Autodesk Fusion 360 part; units mm, degrees
sketch "Skizze1" plane through (0, 0, 0) normal (0, 1, 0) x (1, 0, 0)
  circle A0 centre (0, 0) radius 7.1
  dimension "d1" = 14.2
extrude "Extrusion1" add sketch "Skizze1" along normal blind 50.2

Autodesk Fusion 360 part; units mm, degrees
sketch "Skizze1" plane through (0, 0, 0) normal (0, 1, 0) x (1, 0, 0)
  line L0 (-14.5, 9) -> (14.5, 9)
  line L1 (14.5, 9) -> (14.5, -9)
  line L2 (14.5, -9) -> (-14.5, -9)
  line L3 (-14.5, -9) -> (-14.5, 9)
  line L4 (0, 0) -> (0, 9) construction
  line L5 (0, 0) -> (14.5, 0) construction
  dimension "d1" = 29
  dimension "d2" = 18
extrude "Extrusion1" add sketch "Skizze1" along normal blind 4

Autodesk Fusion 360 part; units mm, degrees
sketch "Skizze1" plane through (0, 0, 0) normal (0, 1, 0) x (1, 0, 0)
  line L0 (-15.015, 0) -> (31.025, 0) construction
  line L1 (-15.015, 0) -> (-15.015, -7.62)
  line L2 (-15.015, -7.62) -> (15.015, -7.62)
  line L3 (15.015, -7.62) -> (16.625, -6.01)
  line L4 (16.625, -6.01) -> (31.025, -6.01)
  line L5 (31.025, -6.01) -> (31.025, 0)
  line L6 (-15.015, 0) -> (-15.015, 7.62)
  line L7 (-15.015, 7.62) -> (15.015, 7.62)
  line L8 (15.015, 7.62) -> (16.625, 6.01)
  line L9 (16.625, 6.01) -> (31.025, 6.01)
  line L10 (31.025, 6.01) -> (31.025, 0)
  line L11 (0, 0) -> (0, 7.62) construction
  dimension "d1" = 12.02
  dimension "d2" = 15.24
  dimension "d3" = 30.03
  dimension "d4" = 14.4
  dimension "d5" = 46.04
extrude "Extrusion1" add sketch "Skizze1" along normal blind 3

Autodesk Fusion 360 part; units mm, degrees
sketch "Skizze1" plane through (0, 0, 0) normal (0, 1, 0) x (1, 0, 0)
  line L0 (-17, 17) -> (17, 17)
  line L1 (17, 17) -> (17, -17)
  line L2 (17, -17) -> (-17, -17)
  line L3 (-17, -17) -> (-17, 17)
  line L4 (0, 0) -> (0, 17) construction
  line L5 (0, 0) -> (17, 0) construction
  circle A0 centre (0, 0) radius 2
  circle A1 centre (-14, 14) radius 1.55
  circle A2 centre (14, 14) radius 1.55
  circle A3 centre (-14, -14) radius 1.55
  circle A4 centre (14, -14) radius 1.55
  circle A5 centre (0, 0) radius 5
  circle A6 centre (-13.25, -7.5) radius 1.25
  line L6 (-12, -7.5) -> (-12, 7.5)
  line L7 (-14.5, -7.5) -> (-14.5, 7.5)
  circle A7 centre (-6.5, 7.5) radius 5.5
  circle A8 centre (-6.5, 7.5) radius 8
  line L8 (-9.2839, 15) -> (0, 15)
  line L9 (-8.7913, 12.5) -> (0, 12.5)
  circle A9 centre (6.5, 7.5) radius 8
  circle A10 centre (6.5, 7.5) radius 5.5
  line L10 (8.7913, 12.5) -> (0, 12.5)
  line L11 (9.2839, 15) -> (0, 15)
  line L12 (12, -7.5) -> (12, 7.5)
  line L13 (14.5, -7.5) -> (14.5, 7.5)
  circle A11 centre (13.25, -7.5) radius 1.25
  dimension "d1" = 34
  dimension "d7" = 4
  dimension "d11" = 3.1
  dimension "d12" = 28
  dimension "d13" = 28
  dimension "d14" = 10
  dimension "d17" = 2.5
  dimension "d18" = 2.5
  dimension "d20" = 16
  dimension "d21" = 11
  dimension "d22" = 9.5
  dimension "d23" = 2
  dimension "d24" = 2.5
  dimension "d28" = 9.5
extrude "Extrusion1" add sketch "Skizze1" along normal blind 3 contours L0 L1 L2 L3 | A0 A5 A8 A9 | A0 A5 A8 A9 A10 | A0 A5 A7 A8 A9 | A0 A8 A9 | A5 A9 A10 L12 | A5 L6 A7 A8 | A5 A8 A9 | A9 A10 L10 L11 L12 | A9 L12 L13 A11 | A5 A7 L9 A9 | A5 A7 | L6 A7 A8 L8 L9 | A6 L6 L7 A8 | A5 A8 A10 | A5 A7 A8 A9 A10 | A5 A7 A9 | A5 A10 | A5 A8 A10 L10 | A11 | A6 | A8 A10 | A7 A9 | A9 L11 | A10 L10 | A7 L9 | A8 L8 | A8 A9 A10 L10 | A7 A8 L9 A9 | A8 L8 L9 A9 L10 L11 | A8 L9 A9 L10 picked at (0.0445, 2.311)
fillet "Abrundung1" radius 3 4 edges at (-17, 1.5, -17) (-17, 1.5, 17) (17, 1.5, 17) (17, 1.5, -17)
extrude "Extrusion2" cut sketch "Skizze1" along normal up to surface (3 mm away) contours A9 A10 L10 L11 L12 | A9 L12 L13 A11 | L6 A7 A8 L8 L9 | A6 L6 L7 A8 | A11 | A6 | A10 L10 | A7 L9 | A8 L8 L9 A9 L10 L11
sketch "Skizze2" plane through (0, 0, 0) normal (0, -1, 0) x (1, 0, 0)
  arc A0 (-12, 7.5) -> (-14.5, 7.5) centre (-13.25, 7.5) ccw
  line L0 (-12, 7.5) -> (-12, -7.5)
  arc A1 (-12, -7.5) -> (-8.7913, -12.5) centre (-6.5, -7.5) ccw
  line L1 (-8.7913, -12.5) -> (8.7913, -12.5)
  arc A2 (8.7913, -12.5) -> (12, -7.5) centre (6.5, -7.5) ccw
  line L2 (12, -7.5) -> (12, 7.5)
  arc A3 (14.5, 7.5) -> (12, 7.5) centre (13.25, 7.5) ccw
  line L3 (14.5, 7.5) -> (14.5, -7.5)
  arc A4 (9.2839, -15) -> (14.5, -7.5) centre (6.5, -7.5) ccw
  line L4 (9.2839, -15) -> (-9.2839, -15)
  arc A5 (-14.5, -7.5) -> (-9.2839, -15) centre (-6.5, -7.5) ccw
  line L5 (-14.5, -7.5) -> (-14.5, 7.5)
  circle A6 centre (-14, 14) radius 1.55
  circle A7 centre (14, -14) radius 1.55
  circle A8 centre (14, 14) radius 1.55
  circle A9 centre (-14, -14) radius 1.55
  circle A10 centre (0, 0) radius 2
  arc A11 (14, -17) -> (17, -14) centre (14, -14) ccw
  line L6 (17, -14) -> (17, 14)
  arc A12 (17, 14) -> (14, 17) centre (14, 14) ccw
  line L7 (14, 17) -> (-14, 17)
  arc A13 (-14, 17) -> (-17, 14) centre (-14, 14) ccw
  line L8 (-17, 14) -> (-17, -14)
  arc A14 (-17, -14) -> (-14, -17) centre (-14, -14) ccw
  line L9 (-14, -17) -> (14, -17)
  circle A15 centre (0, 0) radius 5
  line L10 (0, 0) -> (0, -17) construction
  circle A16 centre (6.25, -7.5) radius 1.25
  line L11 (5, 0) -> (5, -7.5)
  line L12 (7.5, -7.5) -> (7.5, 0)
  circle A17 centre (0, 0) radius 7.5
  line L13 (0, 0) -> (7.5, 0) construction
  circle A18 centre (-6.25, -7.5) radius 1.25
  line L14 (-5, 0) -> (-5, -7.5)
  line L15 (-7.5, -7.5) -> (-7.5, 0)
  dimension "d31" = 2.5
  dimension "d32" = 10
  dimension "d33" = 7.5
extrude "Extrusion3" cut sketch "Skizze2" against normal up to surface (3 mm away) contours A15 L11 A17 L14 | A16 L11 L12 A17 | A17 A18 L14 L15 | A16 | A18 picked at (-4.6131, 4.7886)
equation "d13 = d12"
equation "d21 = d20 - 5 mm"
Design review of the part built by this model. Coordinates are the model's own, in mm. A direction names the side the tool comes from. Give positions to 0.01 mm unless a question says otherwise; leave off trailing zeros. Loops run counter-clockwise (first coordinate to the right, second up) from the corner with the lowest first, then second, coordinate; pieces in that order, holes last. Notation, with made-up numbers: M -40,-12 L -3,-12 A11 ccw -3,8 Z; hole C 64,-9 d6. An arc over 180 degrees is marked long. Return JSON: item names as keys, results as strings. Group by question number.
Item 1: Tool access review of faces 5 (the flat face through (7.5, 1, -4)), 6 (the flat face through (-17, 25, 0)), 7 (the flat face through (0, 3, 6)): name each direction out of +Z, -Z, +X, -X, +Y, -Y from which nothing blocks a thin tool from reaching the whole face with its end or side.
Item 2: Insertion check: pin 1 Ø3.5 at (x, z) = (14, -14) entering from +Y. The pin has a flat end and moves straight along its axis. Give the tip position at first contact, or say it passes through.
Item 3: For probe 1 along X at (y, z) = (15, 14); probe 2 along Z at (x, y) = (0, 1.3); probe 3 along X at (y, z) = (43, -2.5), list the stretches that pass through material, from the lowest coordinate up.
Item 4: Mouldability with a two-part tool opening along Z and no side actions: class faces 1 (the flat face through (-7.5, 1, -4)), 2 (the flat face through (-12, 25, 2)), 3 (the cylindrical face through (16.14, 24.75, 16.1)), 4 (the flat face through (-4, 0, 0)) as released by +Z, released by -Z, zero draft, split by the parting line, or undercut.
Item 5: We need section C-C (x = 6.25). Give the boundary of the cut face in (y, z), and give its area (3 significant figures).
Item 6: We need section D-D (x = 11). Give the boundary of the cut face in (y, z), and give its area (3 significant figures).
Item 7: We need section A-A (y = 30.5). Give the boundary of the cut face in (x, z), and give its area (3 significant figures).
Output:
{
 "1": {"face 5": "+Y, -Y", "face 6": "+Z, -Z, -X, +Y, -Y", "face 7": "-Y"},
 "2": {"pin 1": "stops at y = 50.2"},
 "3": {"probe 1": "x = -17 to -15.55, -12.45 to 12.45, 15.55 to 17", "probe 2": "z = -17 to -15, -12.5 to -2, 2 to 5, 7.5 to 17", "probe 3": "x = -17 to -14.5, 14.5 to 17"},
 "4": {"face 1": "undercut", "face 2": "undercut", "face 3": "released by +Z", "face 4": "zero draft"},
 "5": {"outline": "M 0,-17 L 50.2,-17 L 50.2,-15.5 L 3,-15.5 L 3,-15 L 0,-15 Z; M 0,-12.5 L 3,-12.5 L 3,-8.75 L 0,-8.75 Z; M 0,4.15 L 3,4.15 L 3,0.5 L 50.2,0.5 L 50.2,17 L 0,17 Z", "area": "906 mm^2"},
 "6": {"outline": "M 0,-17 L 50.2,-17 L 50.2,-14.11 L 0,-14.11 Z; M 0,-10.66 L 3,-10.66 L 3,-0.89 L 50.2,-0.89 L 50.2,17 L 0,17 Z", "area": "1,070 mm^2"},
 "7": {"outline": "M -17,-14 A3 ccw -14,-17 L 14,-17 A3 ccw 17,-14 L 17,14 A3 ccw 14,17 L -14,17 A3 ccw -17,14 Z; hole C -14,-14 d3.1; hole C -14,14 d3.1; hole M -14.5,-7.5 A8 ccw -3.72,-15 L 3.72,-15 A8 ccw 14.5,-7.5 L 14.5,7.5 A1.25 ccw 12,7.5 L 12,-1.69 A8 ccw 4.99,0.36 A5 ccw -4.99,0.36 A8 ccw -12,-1.69 L -12,7.5 A1.25 ccw -14.5,7.5 Z; hole C 14,-14 d3.1; hole C 14,14 d3.1", "area": "620 mm^2"}
}
